Read the model definition and answer for the solid it produces. Units are mm, in the model's axes. Face numbers are marked on the shaded views. A direction names the side the tool comes from. Round coordinates to 2 decimals unless told otherwise and drop trailing zeros. Order: outer loops, then holes, each group sorted by start corner. A loop starts at its lowest first (then second) coordinate and runs counter-clockwise, first axis right, second up. Notation, with made-up numbers: (5, 24.25) - (41, 24.25) arc R16 ccw to (41, 44.25) - close; hole circle Ø9 at (33.25, 40). An arc over 180 degrees is marked (long way). Answer as a JSON object with one key per item and string values. Group by question number.
Q1. A tool of negligible diameter and unlimited length cuts with its end or side. For the marked faces 1, 2 and 3, from which of +Z, -Z, +X, -X, +Y, -Y can it reach the whole face along a straight path? Write none if from no direction.
Q2. A cutting plane is placed at A-A on y = 0. Determine the outline of the cut face in (x, z), and give its area (3 significant figures).
Q3. A cutting plane is placed at B-B on x = 5. Determine the outline of the cut face in (y, z).
Q4. Given pin 1 Ø10 at (x, z) = (-25, 5) entering from +Y; pin 2 Ø6 at (x, y) = (6, -6.5) entering from +Z; pin 3 Ø4 at (x, z) = (4, 4.5) entering from -Y; pin 4 Ø2 at (x, z) = (-13, -2) entering from +Y, each flat-ended and moving along its own axis, determine where each tip first touches the part or whether it passes through.
Q5. A cutting plane is placed at C-C on x = -5. Determine the outline of the cut face in (y, z), and give its area (3 significant figures).
Q6. Consider line 1 (Y direction, x = -22, z = -4.25); line 2 (X direction, y = -2.75, z = 6); line 3 (Y direction, x = -10, z = -5.5). Determine where each line is inside the solid, lowest interval first.
```python
from build123d import *

# Parameters (mm, degrees)
SKETCH_1_W          = 14
SKETCH_1_H          = 7.133094656938376
FILLET_1_R          = 10
CUT_EXTRUDE_1_DEPTH = 14


with BuildPart() as part:
    # 草图1 → 旋转1 (revolve)
    with BuildSketch(Plane(origin=(0, 0, 0), x_dir=(1, 0, 0), z_dir=(0, 1, 0)), mode=Mode.PRIVATE) as revolve_1_sk:
        with Locations((-25.681968733439298, 2.0314918872170904)):
            Rectangle(SKETCH_1_W, SKETCH_1_H)
        Polygon((-18.681968733439298, 5.598039215686279), (-18.681968733439298, -1.535055441252097), (-8.681968733439298, -1.5350554412520978), (-8.681968733439302, 0.5980392156862795), (-8.681968733439302, 7.098039215686279), (-18.681968733439298, 7.098039215686279), align=None)
        Polygon((-8.681968733439302, 0.5980392156862795), (-8.681968733439302, -1.535055441252097), (17.318031266560702, -1.5350554412520978), (17.318031266560705, 0.5980392156862795), align=None)
    revolve(revolve_1_sk.sketch.rotate(Axis((-32.6819687334393, 0, 1.5350554412520978), (1, 0, 0)), 180), axis=Axis((-32.6819687334393, 0, 1.5350554412520978), (1, 0, 0)))

    # 圆角1
    # the kernel refuses this fillet: 10 mm, written as the material it adds along each edge
    with BuildSketch(Plane(origin=(-8.681968733439302, 0, 1.5350554412520978), x_dir=(0, 1.2e-16, 1), z_dir=(0, 1, -1.2e-16))) as fillet_1_piece_1:
        with BuildLine():
            CenterArc((12.133094656938377, 9.367496997597598), FILLET_1_R, 180, 69.51268488527734)
            Line((2.1330946569383773, 9.367496997597598), (1.9330946569383771, 9.367496997597598))
            Line((1.9330946569383771, 9.367496997597598), (1.9330946569383771, 0))
            Line((1.9330946569383771, 0), (2.1330946569383773, -0.1999999999999993))
            ThreePointArc((2.1330946569383773, -0.1999999999999993), (5.383094656938376, -0.1999999999999993), (8.563094656938375, -0.18734993995195026))
            Line((8.563094656938375, -0.18734993995195026), (8.633094656938376, 1.78e-15))
        make_face()
    revolve(axis=Axis((-8.681968733439302, 0, 1.5350554412520978), (1, 0, 0)))

    # 草图2 → 切除-拉伸-薄壁1 (cut)
    with BuildSketch(Plane.ZY.offset(32.6819687334393)):
        Polygon((5.514998964205359, 5.919551413658403), (7.454606854910501, 3.979943522953262), (14.525674666775975, 11.051011334818739), (12.586066776070833, 12.99061922552388), align=None)
    extrude(amount=-CUT_EXTRUDE_1_DEPTH, mode=Mode.SUBTRACT)


solid = part.part
```
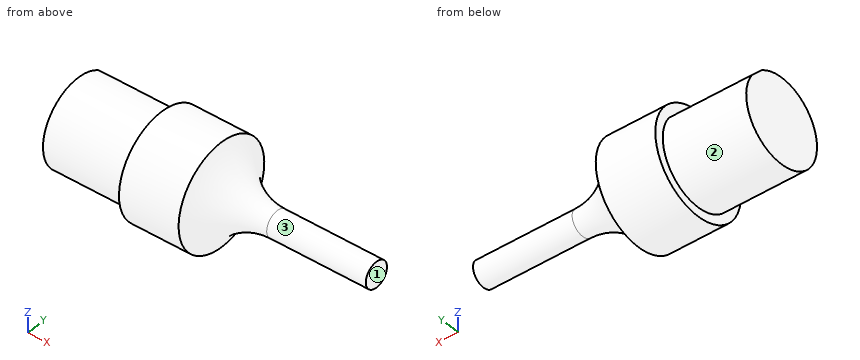
Result set:
{
 "1": {"face 1": "+Z, -Z, +X, +Y, -Y", "face 2": "-X", "face 3": "+X"},
 "2": {"outline": "(-32.68, -5.6) - (-18.68, -5.6) - (-18.68, -7.1) - (-8.68, -7.1) arc R10 cw to (0.69, -0.6) - (17.32, -0.6) - (17.32, 3.67) - (0.69, 3.67) arc R10 cw to (-8.68, 10.17) - (-18.68, 10.17) - (-18.68, 8.67) - (-32.68, 8.67) - close", "area": "517 mm²"},
 "3": {"outline": "circle Ø4.27 at (0, 1.54)"},
 "4": {"pin 1": "stops at y = 7.13", "pin 2": "passes through", "pin 3": "stops at y = -1.9", "pin 4": "stops at y = 8.25"},
 "5": {"outline": "circle Ø7.81 at (0, 1.54)", "area": "47.9 mm²"},
 "6": {"line 1": "y = -4.17 to 4.17", "line 2": "x = -32.68 to -6.56", "line 3": "y = -5 to 5"}
}
